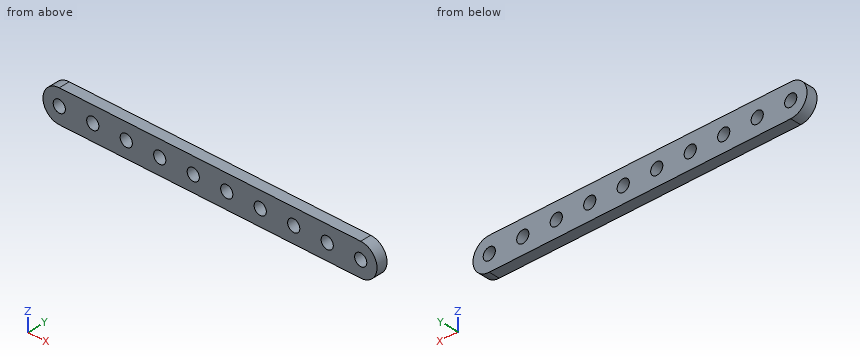
from build123d import *

# Parameters (mm, degrees)
SKETCH1_R           = 1.778
BOSS_EXTRUDE1_DEPTH = 6.35
CUT_EXTRUDE1_DEPTH  = 55.241416026
SKETCH3_W           = 123.961526382
SKETCH3_H           = 57.130094768
CUT_EXTRUDE2_DEPTH  = 3.175


with BuildPart() as part:
    # Sketch1 → Boss-Extrude1 (new body)
    with BuildSketch(Plane.XZ):
        with BuildLine():
            Line((-48.895, -4.7625), (48.895, -4.7625))
            ThreePointArc((48.895, -4.7625), (53.6575, 0), (48.895, 4.7625))
            Line((48.895, 4.7625), (-48.895, 4.7625))
            ThreePointArc((-48.895, 4.7625), (-53.6575, 0), (-48.895, -4.7625))
        make_face()
        with Locations(Location((48.895, 0, 0), (0, 0, 270))):
            Circle(SKETCH1_R, mode=Mode.SUBTRACT)
        with Locations(Location((39.116, 0, 0), (0, 0, 270))):
            Circle(SKETCH1_R, mode=Mode.SUBTRACT)
        with Locations(Location((29.337, 0, 0), (0, 0, 270))):
            Circle(SKETCH1_R, mode=Mode.SUBTRACT)
        with Locations(Location((19.558, 0, 0), (0, 0, 270))):
            Circle(SKETCH1_R, mode=Mode.SUBTRACT)
        with Locations(Location((9.779, 0, 0), (0, 0, 270))):
            Circle(SKETCH1_R, mode=Mode.SUBTRACT)
        with Locations(Location((0, 0, 0), (0, 0, 270))):
            Circle(SKETCH1_R, mode=Mode.SUBTRACT)
        with Locations(Location((-9.779, 0, 0), (0, 0, 270))):
            Circle(SKETCH1_R, mode=Mode.SUBTRACT)
        with Locations(Location((-19.558, 0, 0), (0, 0, 270))):
            Circle(SKETCH1_R, mode=Mode.SUBTRACT)
        with Locations(Location((-29.337, 0, 0), (0, 0, 270))):
            Circle(SKETCH1_R, mode=Mode.SUBTRACT)
        with Locations(Location((-39.116, 0, 0), (0, 0, 270))):
            Circle(SKETCH1_R, mode=Mode.SUBTRACT)
        with Locations(Location((-48.895, 0, 0), (0, 0, 270))):
            Circle(SKETCH1_R, mode=Mode.SUBTRACT)
    extrude(amount=-BOSS_EXTRUDE1_DEPTH)

    # Sketch2 → Cut-Extrude1 (cut, through all)
    with BuildSketch(Plane(origin=(0, 6.35, 0), x_dir=(1, 0, 0), z_dir=(0, 1, 0))):
        with BuildLine():
            Line((-39.116, -4.7625), (-55.615088879, -6.941351058))
            Line((-55.615088879, -6.941351058), (-55.615088879, 8.998214698))
            Line((-55.615088879, 8.998214698), (-39.116, 4.7625))
            ThreePointArc((-39.116, 4.7625), (-43.8785, 0), (-39.116, -4.7625))
        make_face()
    extrude(amount=-CUT_EXTRUDE1_DEPTH, mode=Mode.SUBTRACT)

    # Sketch3 → Cut-Extrude2 (cut)
    with BuildSketch(Plane(origin=(0, 6.35, 0), x_dir=(1, 0, 0), z_dir=(0, 1, 0))):
        with Locations((1.520980261, -5.389631582)):
            Rectangle(SKETCH3_W, SKETCH3_H)
    extrude(amount=-CUT_EXTRUDE2_DEPTH, mode=Mode.SUBTRACT)


solid = part.part
Can you work these out from the model? Positions are in its coordinate system, mm. Coordinates: 2 decimals unless noted, no trailing zeros. Order: outer loops, then holes, each group sorted by start corner. A loop starts at its lowest first (then second) coordinate and runs counter-clockwise, first axis right, second up. Notation, with made-up numbers: (38, -15) - (90, -15) arc R25 cw to (90, 9) - close; hole circle Ø1 at (9.5, 15). An arc over 180 degrees is marked (long way). Answer as a JSON object with one key per item and string values. Group by question number.
Q1. Imagine slicing it at D-D (z = -3.75). Please give me the cut outline in (x, y) (3 decimals).
Q2. Imagine slicing it at B-B (z = 0). Give the number of separate pieces and of enclosed holes in the cut face, and give its area (3 significant figures).
Q3. I need wall thicknesses on line 1 (Z direction, x = 0.5, y = 2); line 2 (Z direction, x = -20.5, y = 2.65); line 3 (X direction, y = 2.9, z = 4.25). Which ranges of each line are inside material? Lowest first, please. Write a range as from..to.
Q4. Imagine slicing it at A-A (x = 0). Please give me the cut outline in (y, z) (1 decimal).
Determined:
{
 "1": {"outline": "(-42.052, 0) - (51.831, 0) - (51.831, 3.175) - (-42.052, 3.175) - close"},
 "2": {"separate pieces": "11", "enclosed holes": "0", "area": "197 mm2"},
 "3": {"line 1": "z = -4.76..-1.71, 1.71..4.76", "line 2": "z = -4.76..-1.51, 1.51..4.76", "line 3": "x = -41.27..51.04"},
 "4": {"outline": "(0, -4.8) - (3.2, -4.8) - (3.2, -1.8) - (0, -1.8) - close; (0, 1.8) - (3.2, 1.8) - (3.2, 4.8) - (0, 4.8) - close"}
}
